The listing builds one solid part. Answer for the finished solid, in the listing's coordinates (mm). A direction names the side the tool comes from. Round coordinates to 2 decimals unless told otherwise and drop trailing zeros. Order: outer loops, then holes, each group sorted by start corner. A loop starts at its lowest first (then second) coordinate and runs counter-clockwise, first axis right, second up. Notation, with made-up numbers: (-30.5, 76) -> (8.5, 76) arc R12 cw to (8.5, 88) -> close; hole circle Ø10 at (-34, -7). An arc over 180 degrees is marked (long way). Return JSON: item names as keys, results as strings. Group by question number.
(1) The part is cut by section C-C (x = 8). Determine the outline of the cut face in (y, z), plus the area to 3 significant figures.
(2) Each of these flat-tipped pins is pushed along its axis until it touches: pin 1 (1.5 mm diameter, centred on y = 0, z = -2, fed in from +X); pin 2 (0.9 mm diameter, centred on y = -1, z = -2, fed in from -X); pin 3 (1.5 mm diameter, centred on x = 17.5, z = -1, fed in from -Y). Where does it stop, or does it pass through?
(3) Which of the six approach directions +Z, -Z, +X, -X, +Y, -Y give full straight-line access (tool end or side, diameter ignored) to faces 5 (the face through (0, 10, 0)), 6 (the face through (-11.5, -4.3, 0.5)), 7 (the face through (-5, 0, -1)), 8 (the face through (-21.162, 6.517, -2.26)), 9 (the face through (21.16, 6.88, -0.23))?
(4) The part is cut by section D-D (x = 18). Determine the outline of the cut face in (y, z).
(5) Consider line 1 (X direction, y = 6.25, z = -3.6); line 2 (Y direction, x = 21.5, z = -2); line 3 (X direction, y = 5.75, z = -0.9). Determine where each line is inside the solid, lowest interval first. Write a range as [from, to].
(6) The part is cut by section A-A (y = 11.5). Determine the outline of the cut face in (x, z).
(7) Determine the mould class of faces 1 (the face through (21.162, 6.517, -1.74)), 2 (the face through (0, 9.5, -1)), 3 (the face through (-7, 10, -3)), 4 (the face through (14.43, 13.9, -1.96)) for opening direction X: +X half, -X half, draft (parallel to the pull), parting line (faces both ways), or undercut.
Autodesk Inventor part; units mm, degrees
ref_plane "YZ Plane" through (0, 0, 0) normal (1, 0, 0) x (0, 1, 0)
ref_plane "XZ Plane" through (0, 0, 0) normal (0, 1, 0) x (-1, 0, 0)
ref_plane "XY Plane" through (0, 0, 0) normal (0, 0, 1) x (1, 0, 0)
sketch "Sketch2" plane through (0, 0, 0) normal (0, 0, 1) x (1, 0, 0)
  line L0 (11.5, -10.5) -> (-11.5, -10.5)
  line L1 (-11.5, -10.5) -> (-11.5, 10.5)
  line L2 (-11.5, 10.5) -> (11.5, 10.5)
  line L3 (11.5, 10.5) -> (11.5, -10.5)
  line L4 (11.5, -10.5) -> (-11.5, 10.5) construction
  line L5 (-11.5, -10.5) -> (11.5, 10.5) construction
  point P0 (0, 0)
  dimension "d0" = 23
  dimension "d1" = 21
extrude "Extrusion1" add sketch "Sketch2" along normal blind 1
sketch "Sketch3" plane through (0, 0, 1) normal (0, 0, 1) x (1, 0, 0)
  line L0 (-7, 14.5) -> (-13, 14.5)
  line L1 (-15, 12.5) -> (-15, 2)
  line L2 (-15, 2) -> (-7, 2)
  line L3 (-7, 2) -> (-7, 14.5)
  line L4 (7, 14.5) -> (13, 14.5)
  line L5 (15, 12.5) -> (15, 2)
  line L6 (15, 2) -> (7, 2)
  line L7 (7, 2) -> (7, 14.5)
  line L8 (-7, 14.5) -> (7, 14.5) construction
  line L9 (0, 14.5) -> (0, 0) construction
  arc A0 (-13, 14.5) -> (-15, 12.5) centre (-13, 12.5) ccw
  arc A1 (15, 12.5) -> (13, 14.5) centre (13, 12.5) ccw
  line L10 (11.5, -10.5) -> (-11.5, -10.5)
  dimension "d5" = 14
  dimension "d6" = 8
  dimension "d7" = 8
  dimension "d9" = 12.5
  dimension "d10" = 2
  dimension "d20" = 12.5
extrude "Extrusion2" add sketch "Sketch3" against normal blind 6
sketch "Sketch6" plane through (0, 0, 0) normal (0, 0, -1) x (-1, 0, 0)
  line L0 (-7, 9.5) -> (7, 9.5)
  line L1 (7, 9.5) -> (7, 2)
  line L2 (7, 2) -> (-7, 2)
  line L3 (-7, 2) -> (-7, 9.5)
  line L4 (-5, 2) -> (5, 2)
  line L5 (5, 2) -> (5, -2)
  line L6 (5, -2) -> (-5, -2)
  line L7 (-5, -2) -> (-5, 2)
  line L8 (-7, 10.5) -> (-7, 2)
  line L9 (7, 10.5) -> (-7, 10.5)
  point P0 (0, 0)
  dimension "d23" = 4
  dimension "d27" = 2
  dimension "d28" = 1
  dimension "d29" = 2
extrude "Extrusion5" add sketch "Sketch6" along normal blind 3
sketch "Sketch4" plane through (15, 2, 1) normal (1, 0, 0) x (0, 0, -1)
  line L0 (0, 10.5) -> (6, 10.5)
  line L1 (3, 10.5) -> (3, 2.5) construction
  circle A0 centre (3, 6.5) radius 2.4
  circle A1 centre (3, 6.5) radius 2
  point P0 (1, -2)
  point P1 (0, 8)
  dimension "d13" = 4.8
  dimension "d14" = 4
  dimension "d15" = 4
extrude "Extrusion3" add sketch "Sketch4" along normal blind 12.5
sketch "Sketch5" plane through (-15, 2, 1) normal (-1, 0, 0) x (0, 0, 1)
  circle A0 centre (-3, 6.5) radius 2.4
  circle A1 centre (-3, 6.5) radius 2
  point P0 (-1, -2)
extrude "Extrusion4" add sketch "Sketch5" along normal blind 12.5
properties part number "flowMeter"
Answer below:
{
 "1": {"outline": "(-10.5, 0) -> (2, 0) -> (2, -5) -> (14.5, -5) -> (14.5, 1) -> (-10.5, 1) -> close", "area": "87.5 mm²"},
 "2": {"pin 1": "stops at x = 5", "pin 2": "stops at x = -5", "pin 3": "stops at y = 6.11"},
 "3": {"face 5": "-Z, +Y", "face 6": "+Z, -Z, -X, -Y", "face 7": "-Z, -X, -Y", "face 8": "-X", "face 9": "+X"},
 "4": {"outline": "circle Ø4.8 at (8.5, -2); hole circle Ø4 at (8.5, -2)"},
 "5": {"line 1": "x = [-15, -7], [7, 15]", "line 2": "y = [6.1, 6.5], [10.5, 10.9]", "line 3": "x = [-15, 15]"},
 "6": {"outline": "(-15, -5) -> (-7, -5) -> (-7, 1) -> (-15, 1) -> close; (7, -5) -> (15, -5) -> (15, 1) -> (7, 1) -> close"},
 "7": {"face 1": "draft", "face 2": "undercut", "face 3": "undercut", "face 4": "+X half"}
}
